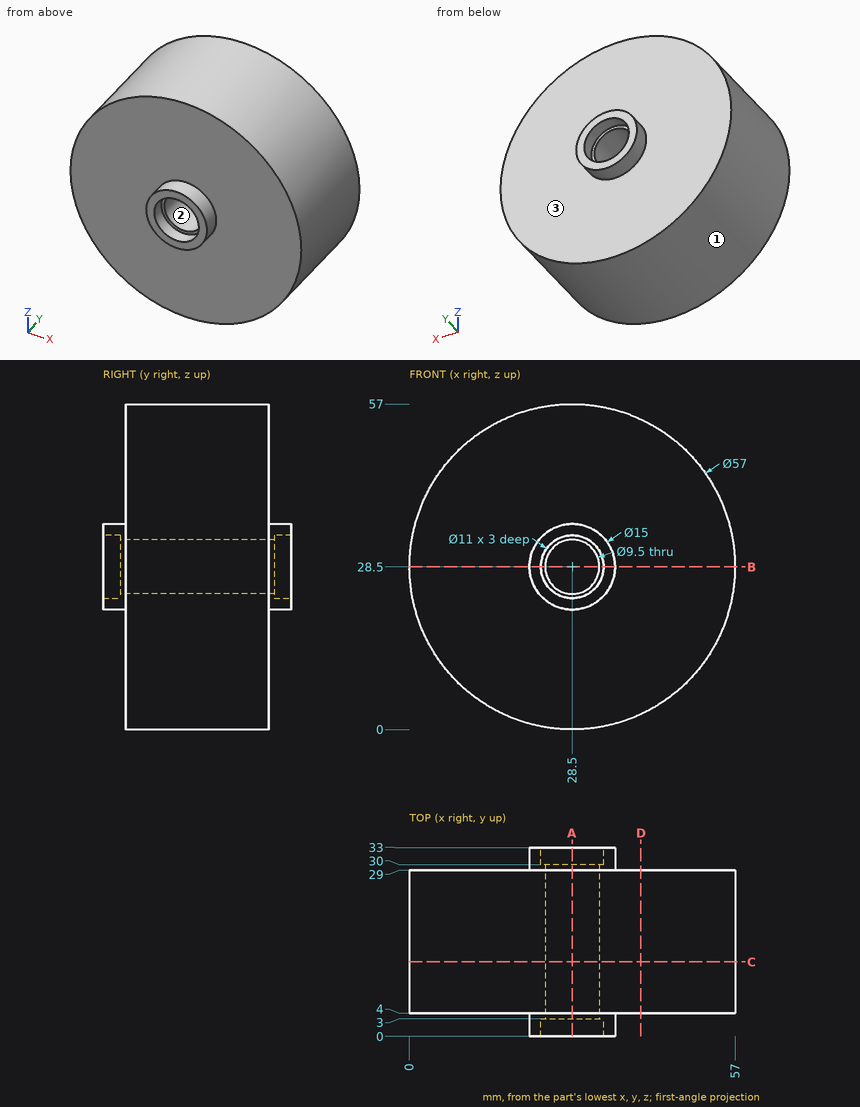
Study the drawing (mm; zero at the part's minimum x, y, z) and answer. Round coordinates to 2 decimals unless told otherwise and drop trailing zeros. Write each loop counter-clockwise with the first axis right and the second up, starting at its lowest first coordinate (ties: lowest second). Pieces come first, ordered by that corner, then holes. Notation, with made-up numbers: (20, 77) - (67, 77) arc R25 cw to (67, 100) - close; hole circle Ø1 at (83, 29.25). An arc over 180 degrees is marked (long way). Return JSON: item names as keys, results as strings. Group by question number.
Q1. The part is cut by section B-B on z = 28.5. Write down the section's boundary in (x, y), then the cut area to 3 significant figures.
Q2. The mould has two halves that part along Z. Classify the marked faces 1, 2 and 3: released by +Z, released by -Z, zero draft, split by the parting line, or undercut.
Q3. The part is cut by section C-C on y = 13. Write down the section's boundary in (x, z), then the cut area to 3 significant figures.
Q4. Find the intervals of material crossed by L1, parallel to X at y = 31.9, z = 28.5; L2, parallel to Y at x = 32.5, z = 53; L3, parallel to X at y = 15, z = 28, in increasing order.
Q5. The part is cut by section A-A on x = 28.5. Write down the section's boundary in (y, z).
Q6. Each of these flat-tipped pins is pushed along its axis until it touches: pin 1 Ø3 at (x, y) = (47.5, 12.5) entering from -Z; pin 2 Ø9 at (x, z) = (30, 26) entering from -Y; pin 3 Ø10 at (x, z) = (28.5, 28.5) entering from -Y; pin 4 Ø1 at (x, y) = (7.5, 14.5) entering from -Z. Where does it stop, or does it pass through?
Q7. The part is cut by section D-D on x = 40.5. Write down the section's boundary in (y, z).
Solved:
{
 "1": {"outline": "(0, 4) - (21, 4) - (21, 0) - (23, 0) - (23, 3) - (23.75, 3) - (23.75, 30) - (23, 30) - (23, 33) - (21, 33) - (21, 29) - (0, 29) - close; (33.25, 3) - (34, 3) - (34, 0) - (36, 0) - (36, 4) - (57, 4) - (57, 29) - (36, 29) - (36, 33) - (34, 33) - (34, 30) - (33.25, 30) - close", "area": "1,220 mm²"},
 "2": {"face 1": "split by the parting line", "face 2": "undercut", "face 3": "zero draft"},
 "3": {"outline": "circle Ø57 at (28.5, 28.5); hole circle Ø9.5 at (28.5, 28.5)", "area": "2,480 mm²"},
 "4": {"L1": "21 to 23, 34 to 36", "L2": "4 to 29", "L3": "0 to 23.78, 33.22 to 57"},
 "5": {"outline": "(0, 21) - (4, 21) - (4, 0) - (29, 0) - (29, 21) - (33, 21) - (33, 23) - (30, 23) - (30, 23.75) - (3, 23.75) - (3, 23) - (0, 23) - close; (0, 34) - (3, 34) - (3, 33.25) - (30, 33.25) - (30, 34) - (33, 34) - (33, 36) - (29, 36) - (29, 57) - (4, 57) - (4, 36) - (0, 36) - close"},
 "6": {"pin 1": "z = 6.01", "pin 2": "y = 0", "pin 3": "y = 3", "pin 4": "z = 8.7"},
 "7": {"outline": "(4, 2.65) - (29, 2.65) - (29, 54.35) - (4, 54.35) - close"}
}
